Design review of the part built by this model. Coordinates are the model's own, in mm. A direction names the side the tool comes from. Give positions to 0.01 mm unless a question says otherwise; leave off trailing zeros. Order: outer loops, then holes, each group sorted by start corner. A loop starts at its lowest first (then second) coordinate and runs counter-clockwise, first axis right, second up. Notation, with made-up numbers: (53.5, 53) -> (91.5, 53) arc R22 cw to (91.5, 66) -> close; hole circle Ø7 at (27.5, 59.5). An arc over 180 degrees is marked (long way). Return JSON: item names as keys, results as strings.
```python
from build123d import *

# Parameters (mm, degrees)
BOSS_EXTRUDE1_DEPTH = 114.3
CUT_EXTRUDE2_DEPTH  = 114.3


with BuildPart() as part:
    # Sketch1 → Boss-Extrude1 (new, symmetric)
    with BuildSketch(Plane(origin=(0, 0, 0), x_dir=(0, 0, -1), z_dir=(1, 0, 0))):
        with BuildLine():
            Line((12.7, 0), (-12.7, 0))
            Line((-12.7, 0), (-12.7, 22.86))
            ThreePointArc((-12.7, 22.86), (-11.956051224, 24.656051224), (-10.16, 25.4))
            Line((-10.16, 25.4), (-1.5875, 25.4))
            Line((-1.5875, 25.4), (-1.5875, 7.62))
            Line((-1.5875, 7.62), (-6.35, 7.62))
            Line((-6.35, 7.62), (-6.35, 2.54))
            Line((-6.35, 2.54), (6.35, 2.54))
            Line((6.35, 2.54), (6.35, 7.62))
            Line((6.35, 7.62), (1.5875, 7.62))
            Line((1.5875, 7.62), (1.5875, 25.4))
            Line((1.5875, 25.4), (10.16, 25.4))
            ThreePointArc((10.16, 25.4), (11.956051224, 24.656051224), (12.7, 22.86))
            Line((12.7, 22.86), (12.7, 0))
        make_face()
    extrude(amount=BOSS_EXTRUDE1_DEPTH, both=True)

    # Sketch2 → Cut-Extrude2 (cut, symmetric)
    with BuildSketch(Plane(origin=(0, 0, 0), x_dir=(0, 0, -1), z_dir=(1, 0, 0))):
        Polygon((-6.35, 7.62), (-1.5875, 12.3825), (-1.5875, 7.62), align=None)
        Polygon((1.5875, 7.62), (6.35, 7.62), (1.5875, 12.3825), align=None)
    extrude(amount=CUT_EXTRUDE2_DEPTH, both=True, mode=Mode.SUBTRACT)


solid = part.part
```
Item 1: Wall thickness on L1, parallel to Z at x = 102, y = 12.75; L2, parallel to Z at x = -81, y = 2.75; L3, parallel to Y at x = -43, z = 0.5: over which ranges is each line inside the solid? List them lowest first. Write a range as [from, to].
Result set:
{"L1": "z = [-12.7, -1.59], [1.59, 12.7]", "L2": "z = [-12.7, -6.35], [6.35, 12.7]", "L3": "y = [0, 2.54]"}
Item 2: Add section B-B (x = -58.5). Give the boundary of the cut face in (y, z), plus the area to 3 significant figures.
Result set:
{"outline": "(0, -12.7) -> (22.86, -12.7) arc R2.54 ccw to (25.4, -10.16) -> (25.4, -1.59) -> (12.38, -1.59) -> (7.62, -6.35) -> (2.54, -6.35) -> (2.54, 6.35) -> (7.62, 6.35) -> (12.38, 1.59) -> (25.4, 1.59) -> (25.4, 10.16) arc R2.54 ccw to (22.86, 12.7) -> (0, 12.7) -> close", "area": "499 mm^2"}
Item 3: Mouldability with a two-part tool opening along Y and no side actions: class faces 4 (the face through (1.6, 9.97, -4)), 5 (the face through (114.3, 13, 3)), 6 (the face through (2, 25.4, 6)) as released by +Y, released by -Y, zero draft, split by the parting line, or undercut.
Result set:
{"face 4": "undercut", "face 5": "zero draft", "face 6": "released by +Y"}
Item 4: For pin 1 (14 mm diameter, centred on x = -30, z = -1.5, fed in from +Y), flat-tipped, find the tip position at first contact; note if it passes through.
Result set:
{"pin 1": "stops at y = 25.4"}
Item 5: Add section A-A (y = 18.75). Give the boundary of the cut face in (x, z).
Result set:
{"outline": "(-114.3, -12.7) -> (114.3, -12.7) -> (114.3, -1.59) -> (-114.3, -1.59) -> close; (-114.3, 1.59) -> (114.3, 1.59) -> (114.3, 12.7) -> (-114.3, 12.7) -> close"}
Item 6: Machinability: for faces 1 (the face through (-114.3, 13, 3)), 2 (the face through (2, 2.54, 0)), 3 (the face through (2, 19, 1.588)), which of the approach directions +Z, -Z, +X, -X, +Y, -Y give a long, thin tool a straight path to every point of the face, cutting with its end or side? Answer none if there is none.
Result set:
{"face 1": "+Z, -Z, -X, +Y, -Y", "face 2": "+X, -X", "face 3": "+X, -X, +Y"}
